```python
from build123d import *

# Parameters (mm, degrees)
F0_R     = 46.8986478897
F1_DEPTH = 25
F2_DEPTH = 53
F3_R     = 33.7989898732


with BuildPart() as f1:
    # F0 (on Top) → F1 (new body)
    with BuildSketch(Plane.XY):
        with Locations((0, 9.0647488832)):
            Circle(F0_R)
    extrude(amount=F1_DEPTH)

    # F2 (add): a face of the model
    f2_faces = [f1.faces().sort_by_distance(p)[0] for p in [
        (0, 9.0647488832, 25),
    ]]
    extrude(f2_faces, amount=F2_DEPTH)

    # F3
    f3_edges = [f1.edges().sort_by_distance(p)[0] for p in [
        (-46.898648, 9.064749, 78),
    ]]
    fillet(f3_edges, radius=F3_R)


solid = f1.part
```
Verification items for the finished model (mm, model axes). Give positions to 0.01 mm unless a question says otherwise; leave off trailing zeros. Loops run counter-clockwise (first coordinate to the right, second up) from the corner with the lowest first, then second, coordinate; pieces in that order, holes last.
1. Thickness scan on line 1 (Z direction, x = 29.5, y = 20); line 2 (Y direction, x = 29, z = 53); line 3 (Y direction, x = 29, z = 37.5). Record the ranges inside material, lowest first.
2. Section check A-A, the plane z = 33. Enter the section's corners in (x, y), then the cut area to 3 significant figures.
3. Go/stop test with flat-tipped pins: pin 1 Ø6 at (y, z) = (22, 20) entering from +X; pin 2 Ø2 at (x, z) = (-21, 10.5) entering from +Y; pin 3 Ø1.5 at (y, z) = (25, 32) entering from +X. Record where each tip stops, or that it passes through.
Geometry says:
1. line 1: z = 0 to 72.58
1. line 2: y = -26.3 to 44.43
1. line 3: y = -27.79 to 45.92
2. outline: circle Ø93.8 at (0, 9.06)
2. area: 6,910 mm2
3. pin 1: stops at x = 45.83
3. pin 2: stops at y = 51.49
3. pin 3: stops at x = 44.37
